from build123d import *

# Parameters (mm, degrees)
BOSS_EXTRUDE1_DEPTH = 5
SKETCH5_R           = 2.5
CUT_EXTRUDE3_DEPTH  = 10
FILLET2_R           = 2
SKETCH6_R           = 1.5
CUT_EXTRUDE5_DEPTH  = 10
SKETCH7_W           = 3.604584819
SKETCH7_H           = 28.321717567
CUT_EXTRUDE6_DEPTH  = 10
SKETCH8_R           = 1.5
SKETCH8_R_2         = 1.459602963
CUT_EXTRUDE7_DEPTH  = 10


with BuildPart() as part:
    # Sketch1 → Boss-Extrude1 (new body)
    with BuildSketch(Plane(origin=(0, 0, 0), x_dir=(1, 0, 0), z_dir=(0, 1, 0))):
        Polygon((-12.452830189, 99.902137597), (37.547169811, 149.902137597), (67.547169811, 149.902137597), (67.547169811, 129.902137597), (147.547169811, 129.902137597), (147.547169811, 149.902137597), (187.547169811, 149.902137597), (187.547169811, -50.097862403), (147.547169811, -50.097862403), (147.547169811, -30.097862403), (67.547169811, -30.097862403), (67.547169811, -50.097862403), (37.547169811, -50.097862403), (-12.452830189, -0.097862403), align=None)
    extrude(amount=BOSS_EXTRUDE1_DEPTH)

    # Sketch5 → Cut-Extrude3 (cut)
    with BuildSketch(Plane(origin=(0, 5, 0), x_dir=(1, 0, 0), z_dir=(0, 1, 0))):
        with Locations(Location((178.627103709, 49.902137597, 0), (0, 0, 270))):
            Circle(SKETCH5_R)
    extrude(amount=-CUT_EXTRUDE3_DEPTH, mode=Mode.SUBTRACT)

    # Fillet2
    fillet2_edges = [part.edges().sort_by_distance(p)[0] for p in [
        (-12.452830189, 2.5, -99.902137597),
        (37.547169811, 2.5, -149.902137597),
        (67.547169811, 2.5, -149.902137597),
        (147.547169811, 2.5, -149.902137597),
        (187.547169811, 2.5, -149.902137597),
        (187.547169811, 2.5, 50.097862403),
        (147.547169811, 2.5, 50.097862403),
        (67.547169811, 2.5, 50.097862403),
        (37.547169811, 2.5, 50.097862403),
        (-12.452830189, 2.5, 0.097862403),
    ]]
    fillet(fillet2_edges, radius=FILLET2_R)

    # Sketch6 → Cut-Extrude5 (cut)
    with BuildSketch(Plane(origin=(0, 5, 0), x_dir=(1, 0, 0), z_dir=(0, 1, 0))):
        with Locations(Location((22.062785461, 14.910780602, 0), (0, 0, 270))):
            Circle(SKETCH6_R)
        with Locations(Location((22.062785461, 84.910780602, 0), (0, 0, 270))):
            Circle(SKETCH6_R)
    extrude(amount=-CUT_EXTRUDE5_DEPTH, mode=Mode.SUBTRACT)

    # Sketch7 → Cut-Extrude6 (cut)
    with BuildSketch(Plane.XZ):
        with Locations((23.760493051, -49.732417236)):
            Rectangle(SKETCH7_W, SKETCH7_H)
    extrude(amount=-CUT_EXTRUDE6_DEPTH, mode=Mode.SUBTRACT)

    # Sketch8 → Cut-Extrude7 (cut)
    with BuildSketch(Plane(origin=(0, 5, 0), x_dir=(1, 0, 0), z_dir=(0, 1, 0))):
        with Locations(Location((44.14258974, 137.585115599, 0), (0, 0, 270))):
            Circle(SKETCH8_R)
        with Locations(Location((57.926617395, 137.585115599, 0), (0, 0, 270))):
            Circle(SKETCH8_R)
        with Locations(Location((44.14258974, -38.284805306, 0), (0, 0, 270))):
            Circle(SKETCH8_R_2)
        with Locations(Location((57.926617395, -38.284805306, 0), (0, 0, 270))):
            Circle(SKETCH8_R)
        with Locations(Location((156.920997826, -38.284805306, 0), (0, 0, 270))):
            Circle(SKETCH8_R)
        with Locations(Location((176.030672529, -38.284805306, 0), (0, 0, 270))):
            Circle(SKETCH8_R)
        with Locations(Location((156.920997826, 137.585115599, 0), (0, 0, 270))):
            Circle(SKETCH8_R)
        with Locations(Location((176.030672529, 137.585115599, 0), (0, 0, 270))):
            Circle(SKETCH8_R)
    extrude(amount=-CUT_EXTRUDE7_DEPTH, mode=Mode.SUBTRACT)


solid = part.part
Source: CAD feature listing. Evaluate the final solid. Frame: model axes, mm. A direction names the side the tool comes from. Coordinates: 2 decimals unless noted, no trailing zeros. Loops run counter-clockwise (first coordinate to the right, second up) from the corner with the lowest first, then second, coordinate; pieces in that order, holes last. Notation, with made-up numbers: (31.5, 33) - (35.5, 33) arc R25 cw to (35.5, 50) - close; hole circle Ø10 at (65.5, 15). An arc over 180 degrees is marked (long way). One line per item, written item: value. Start each with the question number.
1. Ray query, L1, parallel to Z at x = 156.5, y = 1.25; L2, parallel to X at y = 3.1, z = -50; L3, parallel to X at y = 1.05, z = -137.5 (3 decimals). Return the intervals inside material, ascending.
2. Section A-A (z = -133). Return the cut outline in (x, y), and give its area (3 significant figures).
3. Set-up query: faces 4 (the flat face through (108, 2, 30.098)), 5 (the flat face through (25.563, 2, -50)), 6 (the flat face through (67.547, 2, -139)). Return all of +Z, -Z, +X, -X, +Y, -Y with unobstructed straight access to the full face (end or side cutting, diameter ignored); none if empty.
4. Section C-C (y = 1.9). State how many separate pieces and enclosed holes the cut face has, and give its area (3 significant figures).
5. Section B-B (x = 87). Return the cut outline in (y, z), and give its area (3 significant figures).
6. Contact query for flat-ended pins moving along their axis: P1, Ø4, axis at x = 176.03, z = 38.28, coming from the +Y side; P2, Ø2.5, axis at y = 2, z = -138, coming from the -X side; P3, Ø1.1, axis at x = 24, y = 2.5, coming from the -Z side; P4, Ø1, axis at x = 106.5, y = 0.5, coming from the +Z side. Output: stop coordinate, or through.
7. Mould query, pull axis X, two halves, no side actions, for faces 1 (the flat face through (67.547, 2, 39)), 2 (the flat face through (12.205, 2.465, -124.56)), 3 (the flat face through (89, 0, -51)). Classes: pulls with the +X half, pulls with the -X half, needs draft (parallel to the pull), parting line crosses it, or undercut.
8. Section D-D (z = 21.5). Return the cut outline in (x, y), and give its area (3 significant figures).
Verdict:
1. L1: z = -149.9 to -139.02, -136.15 to 36.85, 39.72 to 50.1
1. L2: x = -12.45 to 21.96, 25.56 to 176.13, 181.13 to 187.55
1. L3: x = 25.145 to 42.645, 45.64 to 56.429, 59.424 to 67.547, 147.547 to 155.423, 158.419 to 174.533, 177.528 to 187.547
2. outline: (20.65, 0) - (67.55, 0) - (67.55, 5) - (20.65, 5) - close; (147.55, 0) - (187.55, 0) - (187.55, 5) - (147.55, 5) - close
2. area: 435 mm2
3. face 4: +Z, +Y, -Y
3. face 5: +Y, -Y
3. face 6: -Z, +Y, -Y
4. separate pieces: 1
4. enclosed holes: 12
4. area: 34,100 mm2
5. outline: (0, -129.9) - (5, -129.9) - (5, 30.1) - (0, 30.1) - close
5. area: 800 mm2
6. P1: stops at y = 5
6. P2: stops at x = 24.4
6. P3: stops at z = -136.9
6. P4: stops at z = 30.1
7. face 1: undercut
7. face 2: pulls with the -X half
7. face 3: needs draft
8. outline: (8.95, 0) - (187.55, 0) - (187.55, 5) - (8.95, 5) - close
8. area: 893 mm2
